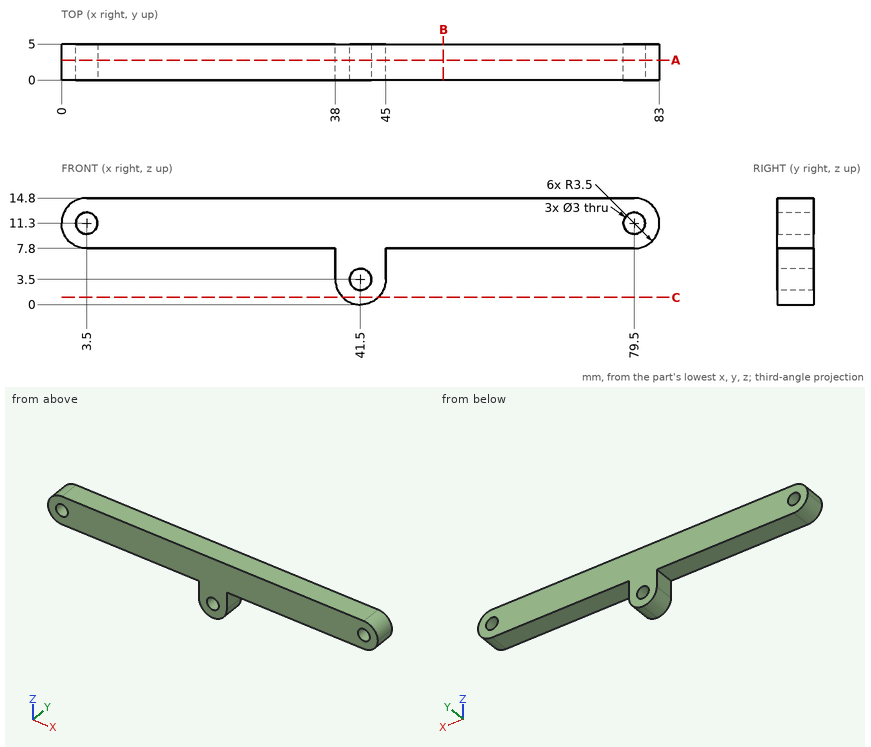
Input: dimensioned drawing with shaded views. Units: mm. Origin: part minimum x, y, z. Round coordinates to 2 decimals unless told otherwise and drop trailing zeros. Loops run counter-clockwise (first coordinate to the right, second up) from the corner with the lowest first, then second, coordinate; pieces in that order, holes last. Notation, with made-up numbers: M 61.25,0 L 72.25,0 A25 cw 72.25,12 Z; hole C -32,53 d4. An arc over 180 degrees is marked long. Return JSON: item names as keys, results as strings. Group by question number.
1. Section query C-C on z = 1. Output: boundary loops of the cut face in (x, y), and give its area (3 significant figures).
2. Section query B-B on x = 53. Output: boundary loops of the cut face in (y, z).
3. Section query A-A on y = 2.75. State how many separate pieces and enclosed holes the cut face has, and give its area (3 significant figures).
4. Pin query (flat end, axial travel): pin 1 (3 mm diameter, centred on y = 1.5, z = 3.5, fed in from -X); pin 2 (1.5 mm diameter, centred on x = 10.5, y = 2, fed in from -Z); pin 3 (2.5 mm diameter, centred on x = 79.5, z = 11.3, fed in from -Y). Return the tip coordinate at first contact, or that it passes through.
5. Material intervals for line 1 along X through (y, z) = (2.9, 11.3); line 2 along Z through (x, y) = (3.5, 3.1); line 3 along X through (y, z) = (4.5, 10.75), sorted ascending. Write a range as from..to.
Checks:
{
 "1": {"outline": "M 39.05,0 L 43.95,0 L 43.95,5 L 39.05,5 Z", "area": "24.5 mm²"},
 "2": {"outline": "M 0,7.8 L 5,7.8 L 5,14.8 L 0,14.8 Z"},
 "3": {"separate pieces": "1", "enclosed holes": "3", "area": "599 mm²"},
 "4": {"pin 1": "stops at x = 38", "pin 2": "stops at z = 7.8", "pin 3": "passes through"},
 "5": {"line 1": "x = 0..2, 5..78, 81..83", "line 2": "z = 7.8..9.8, 12.8..14.8", "line 3": "x = 0.04..2.1, 4.9..78.1, 80.9..82.96"}
}
